Source: three-view drawing plus pictorial views. Frame: mm from the lowest corner of the part. Give positions to 0.01 mm unless a question says otherwise; leave off trailing zeros. Write each loop counter-clockwise with the first axis right and the second up, starting at its lowest first coordinate (ties: lowest second). Pieces come first, ordered by that corner, then holes. Notation, with made-up numbers: (86.5, 51.5) -> (112.5, 51.5) arc R27 ccw to (112.5, 82.5) -> close; hole circle Ø6 at (-12.75, 2). An arc over 180 degrees is marked (long way). Write item = value, one per line.
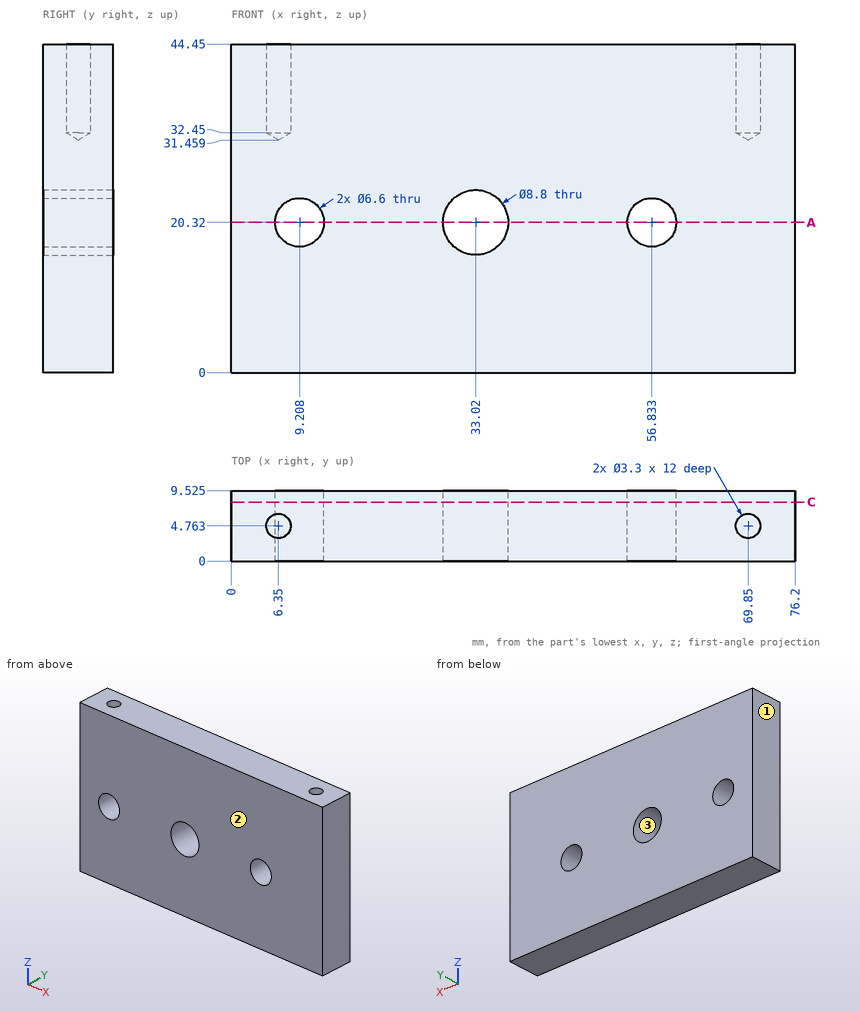
1) Cut plane A-A (z = 20.32). Return the cut outline in (x, y) (1 decimal).
Computed:
outline = (0, 0) -> (5.9, 0) -> (5.9, 9.5) -> (0, 9.5) -> close; (12.5, 0) -> (28.6, 0) -> (28.6, 9.5) -> (12.5, 9.5) -> close; (37.4, 0) -> (53.5, 0) -> (53.5, 9.5) -> (37.4, 9.5) -> close; (60.1, 0) -> (76.2, 0) -> (76.2, 9.5) -> (60.1, 9.5) -> close
2) Contact query for a flat-ended pin moving along its axis: pin 1 (2.5 mm diameter, centred on x = 69.85, y = 4.76, fed in from +Z). Output: stop coordinate, or through.
Computed:
pin_1 = 32.21
3) Draft query along X for the marked faces 1, 2 and 3. Return one class per face: pulls with the +X half, pulls with the -X half, needs draft (parallel to the pull), parting line crosses it, or undercut.
Computed:
face_1 = pulls with the -X half
face_2 = needs draft
face_3 = undercut
4) Material intervals for L1, parallel to Z at x = 33.02, y = 5.75; L2, parallel to X at y = 3, z = 19; L3, parallel to Y at x = 69.85, z = 41 (1 decimal), sorted ascending.
Computed:
L1 = 0 to 15.92, 24.72 to 44.45
L2 = 0 to 6.18, 12.23 to 28.82, 37.22 to 53.81, 59.86 to 76.2
L3 = 0 to 3.1, 6.4 to 9.5
5) Cut plane C-C (y = 8). Return the cut outline in (x, z).
Computed:
outline = (0, 0) -> (76.2, 0) -> (76.2, 44.45) -> (0, 44.45) -> close; hole circle Ø6.6 at (9.21, 20.32); hole circle Ø8.8 at (33.02, 20.32); hole circle Ø6.6 at (56.83, 20.32)
